Here's how the part is built. I have some questions about the finished solid (model axes, mm). A direction names the side the tool comes from. Give positions to 0.01 mm unless a question says otherwise; leave off trailing zeros. Write each loop counter-clockwise with the first axis right and the second up, starting at its lowest first coordinate (ties: lowest second). Pieces come first, ordered by that corner, then holes. Notation, with made-up numbers: (83.25, 80) -> (118.25, 80) arc R10 cw to (118.25, 93) -> close; hole circle Ø5 at (73, 41.5). An arc over 180 degrees is marked (long way). Return JSON: item names as keys, results as strings.
Autodesk Inventor part; units mm, degrees
ref_plane "YZ Plane" through (0, 0, 0) normal (1, 0, 0) x (0, 1, 0)
ref_plane "XZ Plane" through (0, 0, 0) normal (0, 1, 0) x (-1, 0, 0)
ref_plane "XY Plane" through (0, 0, 0) normal (0, 0, 1) x (1, 0, 0)
sketch "Sketch1" plane through (0, 0, 0) normal (0, 1, 0) x (-1, 0, 0)
  line L0 (-72, 30) -> (72, 30)
  line L1 (72, 30) -> (72, -30)
  line L2 (72, -30) -> (-72, -30)
  line L3 (-72, -30) -> (-72, 30)
  point P0 (0, 0)
  dimension "d0" = 144
  dimension "d1" = 60
  dimension "d2" = 72
  dimension "d3" = 30
extrude "Plate1" add sketch "Sketch1" along normal blind 0.5
sketch "Sketch3" plane through (72, 0.5, -30) normal (1, 0, 0) x (0, 1, 0)
  line L0 (0, 60) -> (0, 0)
  line L1 (0, 0) -> (52.5, 0)
  line L2 (52.5, 0) -> (52.5, 60)
  line L3 (52.5, 60) -> (0, 60)
edge flange "Flange1" height 53 angle 90 thickness 0.5 bend radius 0.5 thickness toward (1, 0, 0) relief tear relief width 0.5 relief depth 0.25 corner gap 0.5 corner form 0 edges at (72, 0.5, 0) (-72, 0.5, 0) wall of the first edge with corners at (72, 0.5, 30) (72, 0.5, -30) (72, 53, -30) (72, 53, 30)
bend "Bend1"
corner "Corner1"
fillet "Corner Round1" radius 5 4 edges at (-72.25, 53, -30) (-72.25, 53, 30) (72.25, 53, -30) (72.25, 53, 30)
sketch "Sketch4" plane through (72.5, 1, 30) normal (1, 0, 0) x (0, 0, -1)
  line L0 (5, 52) -> (55, 52)
  line L1 (60, 47) -> (60, 0)
  line L2 (5.7596, 45.6824) -> (55, 37) construction
  point P0 (30, -1)
  dimension "d19" = 5
  dimension "d20" = 15
  dimension "d21" = 50
  dimension "d22" = 10
hole "Hole1" at (72.5, 38, -25) at (72.5, 46.6824, 24.2404) direction (-1, 0, 0) diameter 4 end through all
equation "\"d28\" = Thickness"
equation "\"d8\" = BendReliefWidth"
equation "\"d9\" = BendReliefDepth"
equation "\"d10\" = MinimumRemnant"
equation "\"d11\" = BendRadius"
equation "\"d14\" = BendRadius"
equation "\"d15\" = CornerReliefSize"
equation "\"d16\" = GapSize"
equation "\"d17\" = JacobiRadiusSize"
equation "\"BendRadius\" = Thickness"
equation "\"BendReliefWidth\" = Thickness"
equation "\"BendReliefDepth\" = 0.5 * Thickness"
equation "\"CornerReliefSize\" = 4 * Thickness"
equation "\"MinimumRemnant\" = 2 * Thickness"
equation "\"TransitionRadius\" = BendRadius"
equation "\"JacobiRadiusSize\" = BendRadius"
equation "\"GapSize\" = Thickness"
equation "\"d4\" = BendRadius"
properties part number "radio_base"
1. Suppose I cut it at B-B, the plane y = 31. List the corners of the cut face in (x, z) for me.
Taken from the geometry:
{"outline": "(-72.5, -30) -> (-72, -30) -> (-72, 30) -> (-72.5, 30) -> close; (72, -30) -> (72.5, -30) -> (72.5, 30) -> (72, 30) -> close"}
2. If I drill on line 1 (X direction, y = 6, z = 21); line 2 (Z direction, x = -72.2, y = 38); line 3 (Y direction, x = -72.2, z = -25), over which ranges is the centre line in solid material (lowest first)? Write a range as [from, to].
Taken from the geometry:
{"line 1": "x = [-72.5, -72], [72, 72.5]", "line 2": "z = [-30, -27], [-23, 30]", "line 3": "y = [0.29, 36], [40, 53]"}
3. For pin 1 Ø8 at (x, z) = (-47.5, 16) entering from +Y, with a flat end and sliding along its axis, tell me the tip position at first contact or that it passes through.
Taken from the geometry:
{"pin 1": "stops at y = 0.5"}
4. Suppose I cut it at D-D, the plane x = -26. List the corners of the cut face in (y, z) for me, and give its area (3 significant figures).
Taken from the geometry:
{"outline": "(0, -30) -> (0.5, -30) -> (0.5, 30) -> (0, 30) -> close", "area": "30.0 mm²"}
5. Which directions (+Z, -Z, +X, -X, +Y, -Y) give clear straight access to the entire face, cutting with the end or side of a thin tool? Please do faces 4 (the face through (-72.25, 51.5, 28.57)), 5 (the face through (1, 0.5, 0)).
Taken from the geometry:
{"face 4": "+Z, +X, -X, +Y", "face 5": "+Z, -Z, +Y"}
6. Suppose I cut it at A-A, the plane y = 38. List the corners of the cut face in (x, z) for me, and give its area (3 significant figures).
Taken from the geometry:
{"outline": "(-72.5, -30) -> (-72, -30) -> (-72, -27) -> (-72.5, -27) -> close; (-72.5, -23) -> (-72, -23) -> (-72, 30) -> (-72.5, 30) -> close; (72, -30) -> (72.5, -30) -> (72.5, -27) -> (72, -27) -> close; (72, -23) -> (72.5, -23) -> (72.5, 30) -> (72, 30) -> close", "area": "56.0 mm²"}
7. If we mould it in two halves opening along Z, with no side actions, what happens to faces 1 (the face through (-72, 27, 0)), 2 (the face through (-72.3, 44.7, 24.5)), 3 (the face through (-72.25, 51.57, -28.5))? For each: released by +Z, released by -Z, zero draft, split by the parting line, or undercut.
Taken from the geometry:
{"face 1": "zero draft", "face 2": "undercut", "face 3": "released by -Z"}
8. Suppose I cut it at C-C, the plane z = 12. List the corners of the cut face in (x, y) for me.
Taken from the geometry:
{"outline": "(-72.5, 1) arc R1 ccw to (-71.5, 0) -> (71.5, 0) arc R1 ccw to (72.5, 1) -> (72.5, 53) -> (72, 53) -> (72, 1) arc R0.5 cw to (71.5, 0.5) -> (-71.5, 0.5) arc R0.5 cw to (-72, 1) -> (-72, 53) -> (-72.5, 53) -> close"}
